Could you check a few things on this model? Use its own coordinates, in mm. Face numbers are marked on the shaded views. A direction names the side the tool comes from. Coordinates: 2 decimals unless noted, no trailing zeros. Write each loop counter-clockwise with the first axis right and the second up, starting at its lowest first coordinate (ties: lowest second). Pieces come first, ordered by that corner, then holes.
```python
from build123d import *

# Parameters (mm, degrees)
SKETCH2_R           = 1.25
BOSS_EXTRUDE1_DEPTH = 6.35
SKETCH4_R           = 1.25
CUT_EXTRUDE1_DEPTH  = 17.15


with BuildPart() as part:
    # Sketch2 → Boss-Extrude1 (new body)
    with BuildSketch(Plane(origin=(0, 0, 0), x_dir=(1, 0, 0), z_dir=(0, 1, 0))):
        Polygon((-8.075, 9.816272133), (-5.575, 9.816272133), (-5.575, 3.466272133), (-1.575, 3.466272133), (-1.575, 9.816272133), (1.575, 9.816272133), (1.575, 3.466272133), (5.575, 3.466272133), (5.575, 9.816272133), (8.075, 9.816272133), (8.075, -3.158727867), (-8.075, -3.158727867), align=None)
        with Locations((-3.575, 0)):
            Circle(SKETCH2_R, mode=Mode.SUBTRACT)
        with Locations((3.575, 0)):
            Circle(SKETCH2_R, mode=Mode.SUBTRACT)
    extrude(amount=BOSS_EXTRUDE1_DEPTH)

    # Sketch4 → Cut-Extrude1 (cut, through all)
    with BuildSketch(Plane.ZY.offset(8.075)):
        with Locations((-6.929673598, 3.181098015)):
            Circle(SKETCH4_R)
    extrude(amount=-CUT_EXTRUDE1_DEPTH, mode=Mode.SUBTRACT)


solid = part.part
```
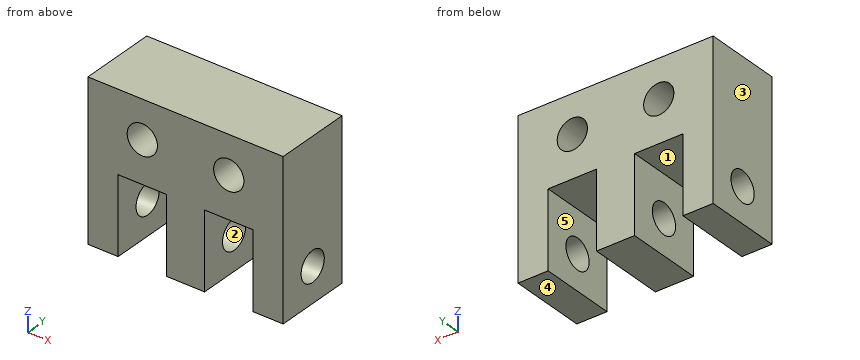
1. I want a section at C-C on x = 3. Please give me the cut outline in (y, z), plus the area to 3 significant figures.
Verdict:
outline: (0, -3.47) - (6.35, -3.47) - (6.35, -1.11) - (0, -1.11) - close; (0, 1.11) - (6.35, 1.11) - (6.35, 3.16) - (0, 3.16) - close
area: 28.0 mm2
2. I want a section at A-A on y = 0.75. Please give me the cut outline in (x, z) (3 decimals).
Verdict:
outline: (-8.075, -9.816) - (-5.575, -9.816) - (-5.575, -3.466) - (-1.575, -3.466) - (-1.575, -9.816) - (1.575, -9.816) - (1.575, -3.466) - (5.575, -3.466) - (5.575, -9.816) - (8.075, -9.816) - (8.075, 3.159) - (-8.075, 3.159) - close; hole circle Ø2.5 at (-3.575, 0); hole circle Ø2.5 at (3.575, 0)
3. On a 3-axis mill with a long thin cutter (end or side, diameter ignored), from which of +Z, -Z, +X, -X, +Y, -Y can I reach the whole of each face in a straight line? I mean the marked faces 1 and 2. Say none if no direction works.
Verdict:
face 1: -Z, +Y, -Y
face 2: +X, -X
4. If we mould it in two halves opening along X, with no side actions, what happens to the marked faces 3, 4 and 5? For each: pulls with the +X half, pulls with the -X half, needs draft (parallel to the pull), parting line crosses it, or undercut.
Verdict:
face 3: pulls with the -X half
face 4: needs draft
face 5: undercut
5. I want a section at D-D on z = 0. Please give me the cut outline in (x, y) (3 decimals).
Verdict:
outline: (-8.075, 0) - (-4.825, 0) - (-4.825, 6.35) - (-8.075, 6.35) - close; (-2.325, 0) - (2.325, 0) - (2.325, 6.35) - (-2.325, 6.35) - close; (4.825, 0) - (8.075, 0) - (8.075, 6.35) - (4.825, 6.35) - close
6. Please list where these lines run through material, in increasing order: line 1 along X through (y, z) = (3, -5) (3 decimals); line 2 along X through (y, z) = (1.75, 0) (3 decimals); line 3 along Z through (x, y) = (1.5, 3.25).
Verdict:
line 1: x = -8.075 to -5.575, -1.575 to 1.575, 5.575 to 8.075
line 2: x = -8.075 to -4.825, -2.325 to 2.325, 4.825 to 8.075
line 3: z = -9.82 to -8.18, -5.68 to 3.16
7. I want a section at B-B on z = -5. Please give me the cut outline in (x, y) (3 decimals), plus the area to 3 significant figures.
Verdict:
outline: (-8.075, 0) - (-5.575, 0) - (-5.575, 6.35) - (-8.075, 6.35) - close; (-1.575, 0) - (1.575, 0) - (1.575, 6.35) - (-1.575, 6.35) - close; (5.575, 0) - (8.075, 0) - (8.075, 6.35) - (5.575, 6.35) - close
area: 51.8 mm2
8. For pin 1 (3 mm diameter, centred on x = 3.575, z = 0, fed in from -Y); pin 2 (1.2 mm diameter, centred on x = -4, y = 4, fed in from -Z), each with a flat end and sliding along its axis, tell me the tip position at first contact or that it passes through.
Verdict:
pin 1: stops at y = 0
pin 2: stops at z = -3.47
